Autodesk Inventor part; units mm, degrees
ref_plane "YZ Plane" through (0, 0, 0) normal (1, 0, 0) x (0, 1, 0)
ref_plane "XZ Plane" through (0, 0, 0) normal (0, 1, 0) x (-1, 0, 0)
ref_plane "XY Plane" through (0, 0, 0) normal (0, 0, 1) x (1, 0, 0)
sketch "Sketch1" plane through (0, 0, 0) normal (0, 0, 1) x (1, 0, 0)
  line L0 (-490, 59) -> (490, 59)
  line L1 (490, 59) -> (490, 0)
  line L2 (490, 0) -> (-490, 0)
  line L3 (-490, 0) -> (-490, 59)
  point P0 (0, 0)
  point P1 (0, 0)
  dimension "d0" = 980
  dimension "d1" = 59
extrude "Plate1" add sketch "Sketch1" along normal blind 2
sketch "Sketch2" plane through (490, -2, 0) normal (0, 1, 0) x (-1, 0, 0)
  line L0 (980, 0) -> (0, 0)
  line L1 (0, 0) -> (0, 20)
  line L2 (0, 20) -> (980, 20)
  line L3 (980, 20) -> (980, 0)
edge flange "Flange1" height 20 angle 90 thickness 2 bend radius 2.75 thickness toward (0, 1, 0) relief round relief width 2 relief depth 1 edges at (0, 0, 2) wall of the first edge with corners at (-490, -2, 0) (490, -2, 0) (490, -2, 20) (-490, -2, 20)
bend "Bend1"
corner "Corner1"
sketch "Sketch5" plane through (0, 0, 0) normal (0, 0, -1) x (-1, 0, 0)
  line L0 (490, 59) -> (-490, 59)
  line L1 (490, -2) -> (-490, -2)
  circle A0 centre (0, 59) radius 17.5
  line L2 (243.4, 59) -> (246.6, 59)
  line L3 (246.6, 59) -> (246.6, 26)
  line L4 (246.6, 26) -> (243.4, 26)
  line L5 (243.4, 26) -> (243.4, 59)
  line L6 (-243.4, 59) -> (-246.6, 59)
  line L7 (-246.6, 59) -> (-246.6, 26)
  line L8 (-246.6, 26) -> (-243.4, 26)
  line L9 (-243.4, 26) -> (-243.4, 59)
  line L10 (0, 59) -> (0, -2) construction
  point P0 (0, 0)
  point P1 (-490, -2)
  point P2 (245, 26)
  point P3 (-245, 26)
  point P4 (246.6, 59)
  point P5 (-17.5, 59)
  point P6 (17.5, 59)
  point P7 (-246.6, 59)
  dimension "d45" = 35
  dimension "d48" = 3.2
  dimension "d49" = 490
  dimension "d51" = 28
  dimension "d52" = 33
extrude "Extrusion1" cut sketch "Sketch5" against normal through all contours L3 L4 L5 L0 | L9 L8 L7 L0 | A0 L0 picked at (-2.238, 52.1497)
sketch "Sketch9" plane through (0, 0, 2) normal (0, 0, 1) x (1, 0, 0)
  line L0 (485.6141, 29.596) -> (485.6141, 17.596) construction
  line L1 (485.6141, 17.596) -> (285.6141, 17.596) construction
  line L2 (285.6141, 17.596) -> (285.6141, 29.596) construction
  line L3 (285.6141, 29.596) -> (485.6141, 29.596) construction
  line L4 (-490, 59) -> (490, 59)
  point P0 (0, 0)
  point P1 (1.05, 68)
  point P2 (490, 59)
  dimension "d40" = 200
  dimension "d41" = 12
mark "Mark2"
equation "\"d2\" = Thickness"
equation "\"d3\" = BendReliefWidth"
equation "\"d4\" = BendReliefDepth"
equation "\"d5\" = MinimumRemnant"
equation "\"d6\" = TransitionRadius"
equation "\"d9\" = BendRadius"
equation "\"d10\" = CornerReliefSize"
equation "\"d11\" = GapSize"
equation "\"d12\" = JacobiRadiusSize"
equation "\"BendReliefWidth\" = Thickness"
equation "\"BendReliefDepth\" = 0.5 * Thickness"
equation "\"CornerReliefSize\" = 4 * Thickness"
equation "\"MinimumRemnant\" = 2 * Thickness"
equation "\"TransitionRadius\" = BendRadius"
equation "\"JacobiRadiusSize\" = BendRadius"
equation "\"GapSize\" = Thickness"
properties part number "MSC 341 stringer BOARD  #" material "Stainless Steel"
Can you work these out from the model? Positions are in its coordinate system, mm. A direction names the side the tool comes from. Round coordinates to 2 decimals unless told otherwise and drop trailing zeros. Order: outer loops, then holes, each group sorted by start corner. A loop starts at its lowest first (then second) coordinate and runs counter-clockwise, first axis right, second up. Notation, with made-up numbers: (51.5, 13.5) -> (86.5, 13.5) arc R20 cw to (86.5, 28.5) -> close; hole circle Ø8 at (27.5, 78). An arc over 180 degrees is marked (long way). Return JSON: item names as keys, results as strings. Group by question number.
1. If we section it at C-C, the plane y = 15: Write out the boundary of the cut face in (x, z).
2. If we section it at D-D, the plane x = 0: Write out the boundary of the cut face in (y, z), then the cut area to 3 significant figures.
3. Which directions (+Z, -Z, +X, -X, +Y, -Y) give clear straight access to the entire face, cutting with the end or side of a thin tool? Please do faces 5 (the face through (-7, 31, 2)), 6 (the face through (-7, 31, 0)).
4. I need wall thicknesses on line 1 (Z direction, x = 349.5, y = 45); line 2 (Y direction, x = -393, z = 10.5); line 3 (Y direction, x = -118.5, z = 4). Which ranges of each line are inside material? Lowest first, please. Write a range as [from, to].
5. We'd pull the mould along X, two halves only. Please class faces 1 (the face through (490, 22, 1)), 2 (the face through (-490, 22, 1)), 3 (the face through (0.385, 41.504, 0.986)), 4 (the face through (7, -2, 12)): released by +X, released by -X, zero draft, split by the parting line, or undercut.
6. If we section it at B-B, the plane z = 9.75: Write out the boundary of the cut face in (x, y), then the cut area to 3 significant figures.
7. Will these pins go through, and if not, where does the flat tip stop? pin 1 (12 mm diameter, centred on x = 169.5, z = 15, fed in from +Y); pin 2 (2 mm diameter, centred on x = -376, y = 32.5, fed in from +Z); pin 3 (10 mm diameter, centred on y = 13, z = 9.5, fed in from -X); pin 4 (1 mm diameter, centred on x = -245.5, z = 0.5, fed in from +Y).
8. If we section it at A-A, the plane x = 306: Write out the boundary of the cut face in (y, z).
Output values:
{
 "1": {"outline": "(-490, 0) -> (490, 0) -> (490, 2) -> (-490, 2) -> close"},
 "2": {"outline": "(-2, 4.75) arc R4.75 ccw to (2.75, 0) -> (41.5, 0) -> (41.5, 2) -> (2.75, 2) arc R2.75 cw to (0, 4.75) -> (0, 20) -> (-2, 20) -> close", "area": "120 mm²"},
 "3": {"face 5": "+Z, +X, -X, +Y", "face 6": "-Z, +X, -X, +Y, -Y"},
 "4": {"line 1": "[0, 2]", "line 2": "[-2, 0]", "line 3": "[-1.94, 0.1]"},
 "5": {"face 1": "released by +X", "face 2": "released by -X", "face 3": "undercut", "face 4": "zero draft"},
 "6": {"outline": "(-490, -2) -> (490, -2) -> (490, 0) -> (-490, 0) -> close", "area": "1,960 mm²"},
 "7": {"pin 1": "y = 0", "pin 2": "z = 2", "pin 3": "through", "pin 4": "y = 26"},
 "8": {"outline": "(-2, 4.75) arc R4.75 ccw to (2.75, 0) -> (59, 0) -> (59, 2) -> (2.75, 2) arc R2.75 cw to (0, 4.75) -> (0, 20) -> (-2, 20) -> close"}
}
